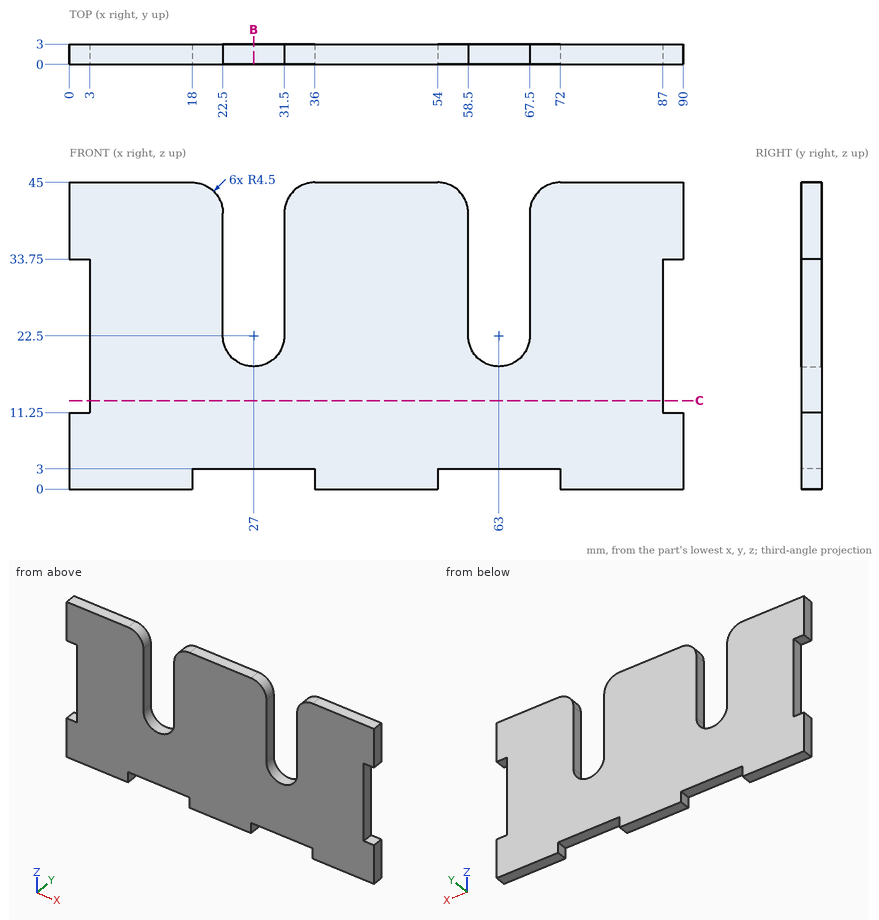
Could you check a few things on this drawing? It's one solid part, dimensions in mm from its lowest x, y, z. Round coordinates to 2 decimals unless told otherwise and drop trailing zeros. Loops run counter-clockwise (first coordinate to the right, second up) from the corner with the lowest first, then second, coordinate; pieces in that order, holes last. Notation, with made-up numbers: (61, 11.5) -> (119, 11.5) arc R24 cw to (119, 35.5) -> close; hole circle Ø2 at (33.25, -22.5). An arc over 180 degrees is marked (long way). One line per item, written item: value. Start each with the question number.
1. For pin 1 (0.9 mm diameter, centred on y = 2, z = 26.5, fed in from -X); pin 2 (1.5 mm diameter, centred on y = 1.5, z = 27.5, fed in from +X); pin 3 (0.9 mm diameter, centred on x = 88, y = 2, fed in from -Z), each with a flat end and sliding along its axis, tell me the tip position at first contact or that it passes through.
2. If we section it at C-C, the plane z = 13: Write out the boundary of the cut face in (x, y).
3. If I drill on probe 1 along X at (y, z) = (1.9, 24); probe 2 along X at (y, z) = (2.6, 37); probe 3 along Z at (x, y) = (64, 2.75), over which ranges is the centre line in solid material (lowest first)?
4. If we section it at B-B, the plane x = 27: Write out the boundary of the cut face in (y, z), then the cut area to 3 significant figures.
Calculated:
1. pin 1: stops at x = 3
1. pin 2: stops at x = 87
1. pin 3: stops at z = 0
2. outline: (3, 0) -> (87, 0) -> (87, 3) -> (3, 3) -> close
3. probe 1: x = 3 to 22.5, 31.5 to 58.5, 67.5 to 87
3. probe 2: x = 0 to 22.5, 31.5 to 58.5, 67.5 to 90
3. probe 3: z = 3 to 18.11
4. outline: (0, 3) -> (3, 3) -> (3, 18) -> (0, 18) -> close
4. area: 45.0 mm²
